Input: part model. Units: mm. Frame: model coordinates. Face numbers are marked on the shaded views. Coordinates: 2 decimals unless noted, no trailing zeros. Write each loop counter-clockwise with the first axis right and the second up, starting at its lowest first coordinate (ties: lowest second). Pieces come first, ordered by that corner, then holes. Notation, with made-up numbers: (79, 66.25) - (110, 66.25) arc R23 ccw to (110, 83.25) - close; hole circle Ø9 at (-19, 15.5). An arc over 180 degrees is marked (long way). Use CSV: the item, a comma, the result in double quotes.
```python
from build123d import *

# Parameters (mm, degrees)
SKETCH2_R           = 57.15
BOSS_EXTRUDE1_DEPTH = 6.35
SKETCH3_R           = 5.15
CUT_EXTRUDE1_DEPTH  = 7.35
CIRPATTERN1_COUNT   = 9
SKETCH6_R           = 1.7
CUT_EXTRUDE4_DEPTH  = 7.35
CIRPATTERN3_COUNT   = 6
SKETCH7_R           = 7.15
SKETCH7_R_2         = 5.15
CUT_EXTRUDE5_DEPTH  = 7.35


with BuildPart() as part:
    # Sketch2 → Boss-Extrude1 (new body)
    with BuildSketch(Plane.XY):
        Circle(SKETCH2_R)
    extrude(amount=BOSS_EXTRUDE1_DEPTH)

    # Sketch3 → Cut-Extrude1 (cut, through all)
    with BuildSketch(Plane.XY.offset(6.35)):
        with Locations((0, 33)):
            Circle(SKETCH3_R)
    cut_extrude1 = extrude(amount=-CUT_EXTRUDE1_DEPTH, mode=Mode.SUBTRACT)

    # CirPattern1: Cut-Extrude1 ×9 about axis
    cirpattern1_axis = Axis((0, 0, 0), (0, 0, 1))
    for i in range(1, CIRPATTERN1_COUNT):
        add(cut_extrude1.rotate(cirpattern1_axis, i * 360 / CIRPATTERN1_COUNT), mode=Mode.SUBTRACT)

    # Sketch6 → Cut-Extrude4 (cut, through all)
    with BuildSketch(Plane.XY.offset(6.35)):
        with Locations((0, 53.975)):
            Circle(SKETCH6_R)
    cut_extrude4 = extrude(amount=-CUT_EXTRUDE4_DEPTH, mode=Mode.SUBTRACT)

    # CirPattern3: Cut-Extrude4 ×6 about axis
    cirpattern3_axis = Axis((0, 0, 0), (0, 0, 1))
    for i in range(1, CIRPATTERN3_COUNT):
        add(cut_extrude4.rotate(cirpattern3_axis, i * 360 / CIRPATTERN3_COUNT), mode=Mode.SUBTRACT)

    # Sketch7 → Cut-Extrude5 (cut, through all)
    with BuildSketch(Plane.XY.offset(6.35)):
        with Locations((-3.616187958, 9.935394759)):
            Circle(SKETCH7_R)
        with Locations((0, -11.752952649)):
            Circle(SKETCH7_R_2)
    extrude(amount=-CUT_EXTRUDE5_DEPTH, mode=Mode.SUBTRACT)


solid = part.part
```
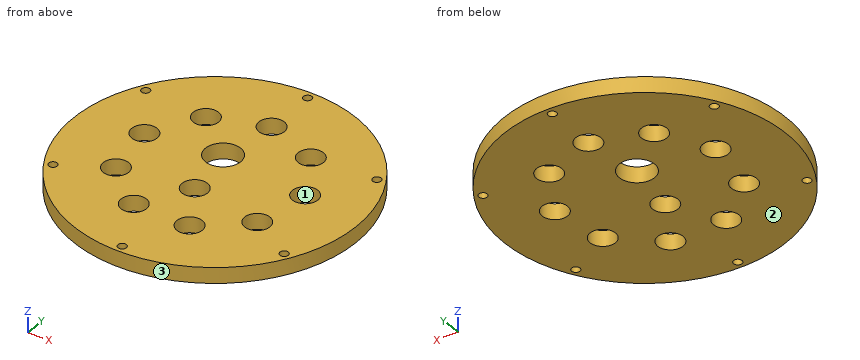
(1) Pin query (flat end, axial travel): pin 1 Ø1.5 at (y, z) = (28, 1) entering from -X; pin 2 Ø2 at (y, z) = (6.5, 5) entering from -X; pin 3 Ø1.5 at (y, z) = (-22, 2.5) entering from +X; pin 4 Ø9.5 at (x, y) = (11.29, -31.01) entering from +Z. Return the tip coordinate at first contact, or that it passes through.
Check values:
pin 1,"x = -50.24"
pin 2,"x = -56.88"
pin 3,"x = 53.05"
pin 4,"through"
(2) Cut plane A-A on y = 8.5. Return loops of the section in (x, z), and give its area (3 significant figures).
Check values:
outline,"(-56.51, 0) - (-36.84, 0) - (-36.84, 6.35) - (-56.51, 6.35) - close; (-28.16, 0) - (-10.62, 0) - (-10.62, 6.35) - (-28.16, 6.35) - close; (3.39, 0) - (28.16, 0) - (28.16, 6.35) - (3.39, 6.35) - close; (36.84, 0) - (56.51, 0) - (56.51, 6.35) - (36.84, 6.35) - close"
area,"518 mm^2"
(3) Cut plane B-B on x = 0. Return loops of the section in (y, z) (3 decimals).
Check values:
outline,"(-57.15, 0) - (-55.675, 0) - (-55.675, 6.35) - (-57.15, 6.35) - close; (-52.275, 0) - (-16.903, 0) - (-16.903, 6.35) - (-52.275, 6.35) - close; (-6.603, 0) - (3.767, 0) - (3.767, 6.35) - (-6.603, 6.35) - close; (16.104, 0) - (27.85, 0) - (27.85, 6.35) - (16.104, 6.35) - close; (38.15, 0) - (52.275, 0) - (52.275, 6.35) - (38.15, 6.35) - close; (55.675, 0) - (57.15, 0) - (57.15, 6.35) - (55.675, 6.35) - close"
(4) Ray query, probe 1 along Y at (x, z) = (1, 3); probe 2 along X at (y, z) = (6, 3.5); probe 3 along X at (y, z) = (21.5, 2.75). Return the intervals inside material, ascending. Write a range as from..to.
Check values:
probe 1,"-57.14..-55.35, -52.6..-16.8, -6.7..4.48, 15.4..27.95, 38.05..52.6, 55.35..57.14"
probe 2,"-56.83..-37.64, -27.36..-9.59, 2.35..27.36, 37.64..56.83"
probe 3,"-52.95..-24.71, -17.71..17.71, 24.71..52.95"
(5) Draft query along Y for the marked faces 1, 2 and 3. Return one class per face: pulls with the +Y half, pulls with the -Y half, needs draft (parallel to the pull), parting line crosses it, or undercut.
Check values:
face 1,"undercut"
face 2,"needs draft"
face 3,"parting line crosses it"
(6) Cut plane C-C on y = 33. Return loops of the section in (x, z).
Check values:
outline,"(-46.66, 0) - (-5.15, 0) - (-5.15, 6.35) - (-46.66, 6.35) - close; (5.15, 0) - (46.66, 0) - (46.66, 6.35) - (5.15, 6.35) - close"
(7) Cut plane D-D on z = 4.25. State how many separate pieces and enclosed holes the cut face has, and give its area (3 significant figures).
Check values:
separate pieces,"1"
enclosed holes,"17"
area,"9,210 mm^2"
